For this review, take the finished solid that the model builds, in its own axes (mm). Face numbers are marked on the shaded views. Round coordinates to 2 decimals unless told otherwise and drop trailing zeros. Write each loop counter-clockwise with the first axis right and the second up, starting at its lowest first coordinate (ties: lowest second). Pieces come first, ordered by that corner, then holes. Notation, with made-up numbers: M 9,61 L 62,61 A35 cw 62,97 Z; hole C 11,62 d7. An arc over 180 degrees is marked long. Write each question's results on one line, items separated by ' | '. Start each with the question number.
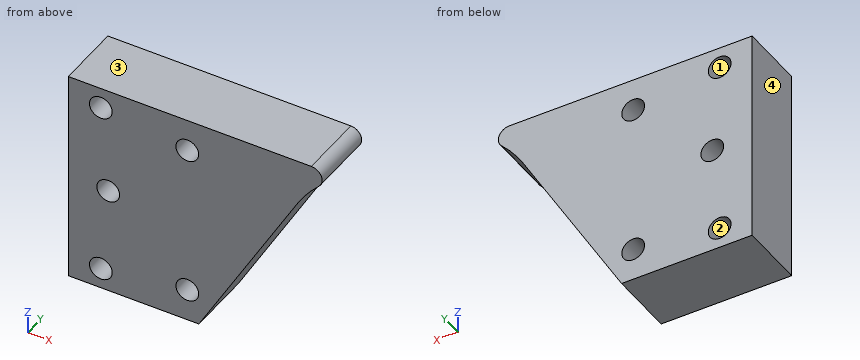
Autodesk Inventor part; units mm, degrees
ref_plane "YZ Plane" through (0, 0, 0) normal (1, 0, 0) x (0, 1, 0)
ref_plane "XZ Plane" through (0, 0, 0) normal (0, 1, 0) x (-1, 0, 0)
ref_plane "XY Plane" through (0, 0, 0) normal (0, 0, 1) x (1, 0, 0)
sketch "Sketch1" plane through (0, 0, 0) normal (0, 1, 0) x (-1, 0, 0)
  line L0 (4, 10) -> (-19.4211, 10)
  line L1 (-19.4211, -10) -> (4, -10)
  line L2 (4, -10) -> (4, 10)
  arc A0 (-19.4211, -10) -> (-19.4211, 10) centre (-25.1, 0) ccw
  line L3 (4, -10) -> (6, -10)
  line L4 (6, -10) -> (6, 10)
  line L5 (6, 10) -> (4, 10)
  line L6 (4, 10) -> (4, -10)
  point P0 (0, 0)
  dimension "d0" = 20
  dimension "d2" = 4
  dimension "d3" = 10
  dimension "d6" = 10
  dimension "d7" = 23
  dimension "d8" = 29.1
  dimension "d11" = 23.4211
  dimension "d12" = 20
  dimension "d13" = 2
extrude "Extrusion1" add sketch "Sketch1" along normal blind 6.07
fillet "Fillet1" radius 1 2 edges at (19.4211, 3.035, 10) (19.4211, 3.035, -10)
sketch "Sketch2" plane through (0, 6.07, 0) normal (0, 1, 0) x (1, 0, 0)
  circle A0 centre (0.68, 0) radius 0.7835
  circle A1 centre (7.98, -7) radius 0.7835
  circle A2 centre (7.98, 7) radius 0.7835
  circle A3 centre (0, -8.07) radius 0.7835
  circle A4 centre (0, 8.07) radius 0.7835
  circle A5 centre (-3, 8.07) radius 1.05
  circle A6 centre (4.98, 7) radius 1.05
  circle A7 centre (-2.32, 0) radius 1.05
  circle A8 centre (4.98, -7) radius 1.05
  circle A9 centre (-3, -8.07) radius 1.05
  point P0 (0, 0)
hole "Hole1" at (4.98, 6.07, 7) at (-2.32, 6.07, 0) at (-3, 6.07, 8.07) at (-3, 6.07, -8.07) at (4.98, 6.07, -7) direction (0, -1, 0) diameter 2.1 depth 7.07
sketch "Sketch3" plane through (0, 0, 0) normal (0, -1, 0) x (1, 0, 0)
  line L0 (18.1137, 10.8993) -> (3.779, -13.929)
  arc A0 (17.1193, 8.28) -> (17.1193, -8.28) centre (25.1, 0) ccw
  line L1 (16.4253, -10) -> (-6, -10)
  arc A1 (16.4253, -10) -> (17.1193, -8.28) centre (16.4253, -9) ccw
  point P0 (0, 0)
  point P1 (15.1407, 5.75)
  point P2 (6.0474, -10)
  dimension "d22" = 60
extrude "Extrusion2" cut sketch "Sketch3" against normal up to next
properties part number "3D_printed_part"
Item 1: We need section B-B on x = -2.32. State the section outline as (y, z) points, then the cut area to 3 significant figures.
Item 2: Insertion check: P1, Ø1.7, axis at x = -3, z = 8.07, coming from the -Y side; P2, Ø2, axis at y = 5, z = -7, coming from the +X side. Each pin has a flat end and moves straight along its axis. Give the tip position at first contact, or say it passes through.
Item 3: We need section A-A on y = 3.75. State the section outline as (x, z) points, then the cut area to 3 significant figures.
Item 4: Mouldability with a two-part tool opening along X and no side actions: class the marked faces 1, 2, 3 and 4 as pulls with the +X half, pulls with the -X half, needs draft (parallel to the pull), parting line crosses it, or undercut.
Item 5: We need section C-C on z = 0.75. State the section outline as (x, y) points, then the cut area to 3 significant figures.
Item 6: We need section D-D on z = -7.5. State the section outline as (x, y) points.
Item 7: For probe 1 along Z at (x, y) = (4.98, 3.75); probe 2 along Z at (x, y) = (-3, 3.75); probe 3 along X at (y, z) = (2, -7.5), list the stretches that pass through material, from the lowest coordinate up.
Numbers:
1) outline: M 0,-10 L 6.07,-10 L 6.07,-8.87 L 0,-8.87 Z; M 0,-7.27 L 6.07,-7.27 L 6.07,-1.05 L 0,-1.05 Z; M 0,1.05 L 6.07,1.05 L 6.07,7.27 L 0,7.27 Z; M 0,8.87 L 6.07,8.87 L 6.07,10 L 0,10 Z | area: 89.2 mm^2
2) P1: passes through | P2: stops at x = 8.36
3) outline: M -6,-10 L 6.05,-10 L 15.14,5.75 A11.5 cw 17.12,8.28 A1 ccw 16.43,10 L -6,10 Z; hole C -3,-8.07 d2.1; hole C -3,8.07 d2.1; hole C -2.32,0 d2.1; hole C 4.98,-7 d2.1; hole C 4.98,7 d2.1 | area: 340 mm^2
4) face 1: undercut | face 2: undercut | face 3: needs draft | face 4: pulls with the -X half
5) outline: M -6,0 L -3.05,0 L -3.05,6.07 L -6,6.07 Z; M -1.59,0 L 12.25,0 L 12.25,6.07 L -1.59,6.07 Z | area: 102 mm^2
6) outline: M -6,0 L -3.88,0 L -3.88,6.07 L -6,6.07 Z; M -2.12,0 L 4.06,0 L 4.06,6.07 L -2.12,6.07 Z; M 5.9,0 L 7.49,0 L 7.49,6.07 L 5.9,6.07 Z
7) probe 1: z = -10 to -8.05, -5.95 to 5.95, 8.05 to 10 | probe 2: z = -10 to -9.12, -7.02 to -0.8, 0.8 to 7.02, 9.12 to 10 | probe 3: x = -6 to -3.88, -2.12 to 4.06, 5.9 to 7.49
